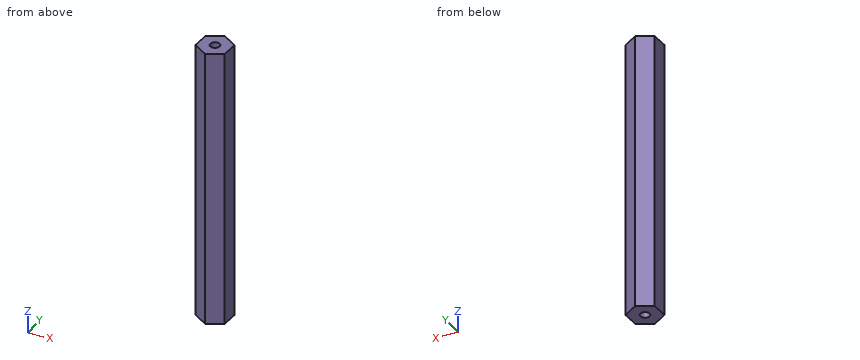
from build123d import *

# Parameters (mm, degrees)
BOSS_EXTRUDE1_DEPTH = 45
SKETCH2_R           = 0.75
CUT_EXTRUDE1_DEPTH  = 5
CUT_EXTRUDE2_START  = -5
SKETCH3_R           = 0.75
CUT_EXTRUDE2_DEPTH  = 5


with BuildPart() as part:
    # Sketch1 → Boss-Extrude1 (new body)
    with BuildSketch(Plane.XY):
        Polygon((2.317732159, -1.480073525), (2.440647352, 1.267178166), (0.122915193, 2.747251691), (-2.317732159, 1.480073525), (-2.440647352, -1.267178166), (-0.122915193, -2.747251691), align=None)
    extrude(amount=BOSS_EXTRUDE1_DEPTH)

    # Sketch2 → Cut-Extrude1 (cut)
    with BuildSketch(Plane.XY.offset(45)):
        Circle(SKETCH2_R)
    extrude(amount=-CUT_EXTRUDE1_DEPTH, mode=Mode.SUBTRACT)

    # Sketch3 → Cut-Extrude2 (cut)
    with BuildSketch(Plane(origin=(0, 0, 0), x_dir=(-1, 0, 0), z_dir=(0, 0, -1)).offset(CUT_EXTRUDE2_START)):
        with Locations(Location((0, 0, 0), (0, 0, 180))):
            Circle(SKETCH3_R)
    extrude(amount=CUT_EXTRUDE2_DEPTH, mode=Mode.SUBTRACT)


solid = part.part
Here's how the part is built. I have some questions about the finished solid (model axes, mm). Round coordinates to 2 decimals unless told otherwise and drop trailing zeros. Loops run counter-clockwise (first coordinate to the right, second up) from the corner with the lowest first, then second, coordinate; pieces in that order, holes last. Notation, with made-up numbers: (36, 6) -> (43, 6) arc R17 cw to (43, 19) -> close; hole circle Ø11 at (33.25, 60.25). An arc over 180 degrees is marked (long way). Write each question's results on one line, items separated by ' | '.
(1) If we section it at B-B, the plane y = 0: List the corners of the cut face in (x, z) for me.
Worked answers:
outline: (-2.38, 0) -> (-0.75, 0) -> (-0.75, 5) -> (0.75, 5) -> (0.75, 0) -> (2.38, 0) -> (2.38, 45) -> (0.75, 45) -> (0.75, 40) -> (-0.75, 40) -> (-0.75, 45) -> (-2.38, 45) -> close
(2) For P1, Ø1.2, axis at x = 0, y = 0, coming from the -Z side; P2, Ø1, axis at y = -0.5, z = 16.5, coming from the -X side, each with a flat end and sliding along its axis, tell me the tip position at first contact or that it passes through.
Worked answers:
P1: z = 5 | P2: x = -2.43
(3) If we section it at C-C, the plane x = 1.6: List the corners of the cut face in (y, z) for me, then the cut area to 3 significant figures.
Worked answers:
outline: (-1.85, 0) -> (1.8, 0) -> (1.8, 45) -> (-1.85, 45) -> close | area: 165 mm2
(4) If I drill on L1, parallel to Z at x = -0.4, y = -0.2; L2, parallel to Y at x = 0, z = 41.4; L3, parallel to Y at x = -0.25, z = 43, over which ranges is the centre line in solid material (lowest first)?
Worked answers:
L1: 5 to 40 | L2: -2.68 to -0.75, 0.75 to 2.68 | L3: -2.67 to -0.71, 0.71 to 2.55
(5) If we section it at D-D, the plane y = -1.9: List the corners of the cut face in (x, z) for me.
Worked answers:
outline: (-1.45, 0) -> (1.51, 0) -> (1.51, 45) -> (-1.45, 45) -> close
(6) If we section it at A-A, the plane z = 23: List the corners of the cut face in (x, y) for me, then the cut area to 3 significant figures.
Worked answers:
outline: (-2.44, -1.27) -> (-0.12, -2.75) -> (2.32, -1.48) -> (2.44, 1.27) -> (0.12, 2.75) -> (-2.32, 1.48) -> close | area: 19.6 mm2
